The listing builds one solid part. Answer for the finished solid, in the listing's coordinates (mm). A direction names the side the tool comes from. Round coordinates to 2 decimals unless told otherwise and drop trailing zeros. Order: outer loops, then holes, each group sorted by start corner. A loop starts at its lowest first (then second) coordinate and runs counter-clockwise, first axis right, second up. Notation, with made-up numbers: (-37, -36.5) - (1, -36.5) arc R22 cw to (1, -15.5) - close; hole circle Ø8 at (15.5, 74). An arc over 180 degrees is marked (long way). Write item = value, one per line.
from build123d import *

# Parameters (mm, degrees)
F0_R     = 6.25
F1_DEPTH = 12.5
F3_DEPTH = 38
F4_R     = 18.99999
F5_R     = 2.5
F6_DEPTH = 5
F7_R     = 7.5
F8_DEPTH = 100


# Not quite as in the source:
# - a fillet or chamfer is up to 0.001 mm smaller than in the source, because OpenCascade refuses the exact size


with BuildPart() as f1:
    # F0 (on Top) → F1 (new body)
    with BuildSketch(Plane.XY):
        with BuildLine():
            Line((-13, 25.5), (-13, 0))
            ThreePointArc((-13, 0), (0, -13), (13, 0))
            Line((13, 0), (13, 13))
            Line((13, 13), (77, 13))
            Line((77, 13), (77, 0))
            ThreePointArc((77, 0), (90, -13), (103, 0))
            Line((103, 0), (103, 64))
            ThreePointArc((103, 64), (90, 77), (77, 64))
            Line((77, 64), (77, 51))
            Line((77, 51), (13, 51))
            Line((13, 51), (13, 64))
            ThreePointArc((13, 64), (0, 77), (-13, 64))
            Line((-13, 64), (-13, 38.5))
            Line((-13, 38.5), (0, 38.5))
            ThreePointArc((0, 38.5), (6.5, 32), (0, 25.5))
            Line((0, 25.5), (-13, 25.5))
        make_face()
        Circle(F0_R, mode=Mode.SUBTRACT)
        with Locations((90, 0)):
            Circle(F0_R, mode=Mode.SUBTRACT)
        with Locations((0, 64)):
            Circle(F0_R, mode=Mode.SUBTRACT)
        with Locations((90, 64)):
            Circle(F0_R, mode=Mode.SUBTRACT)
    extrude(amount=F1_DEPTH)

    # F2 (on face) → F3 (join)
    with BuildSketch(Plane.XZ.offset(-13)):
        Polygon((26.6324676319, 12.5), (77, 12.5), (103, 12.5), (64.8162338159, 50.6837661841), align=None)
    extrude(amount=-F3_DEPTH)

    # F4 (radius 19 in the source; OpenCascade refuses exactly that, so slightly less here)
    f4_edges = [f1.edges().sort_by_distance(p)[0] for p in [
        (45.724351, 13, 31.591883),
        (45.724351, 51, 31.591883),
    ]]
    fillet(f4_edges, radius=F4_R)

    # F5 (on face) → F6 (cut)
    with BuildSketch(Plane(origin=(57.75, 0, 57.75), x_dir=(0.7071067812, 0, -0.7071067812), z_dir=(0.7071067812, 0, 0.7071067812))):
        with Locations((25.1304512677, 20.1117935463)):
            Circle(F5_R)
        with Locations((39.1058761271, 24.6526843463)):
            Circle(F5_R)
        with Locations((39.1058761271, 39.3473156537)):
            Circle(F5_R)
        with Locations((25.1304512677, 43.8882064537)):
            Circle(F5_R)
        with Locations((16.4931636974, 32)):
            Circle(F5_R)
    extrude(amount=-F6_DEPTH, mode=Mode.SUBTRACT)

    # F7 (on face) → F8 (cut)
    with BuildSketch(Plane(origin=(57.75, 0, 57.75), x_dir=(0.7071067812, 0, -0.7071067812), z_dir=(0.7071067812, 0, 0.7071067812))):
        with Locations((28.9931636974, 32)):
            Circle(F7_R)
    extrude(amount=-F8_DEPTH, mode=Mode.SUBTRACT)


solid = f1.part
Q1. For faces 1 (the face through (13, 57, 6)), 2 (the face through (81.84, 39.38, 26.59)), 3 (the face through (6.5, 32.1, 6.2)), determine the directions among +Z, -Z, +X, -X, +Y, -Y from which every point of the face is accessible in a straight line to the end or side of a thin tool.
Model answer:
face_1 = +Z, -Z, +Y
face_2 = none
face_3 = +Z, -Z, -X
Q2. Section B-B on x = 90 is taken. Determine the outline of the cut face in (y, z), then the cut area to 3 significant figures.
Model answer:
outline = (-13, 0) - (-6.25, 0) - (-6.25, 12.5) - (-13, 12.5) - close; (6.25, 0) - (57.75, 0) - (57.75, 12.5) - (51, 12.5) - (51, 25.5) - (13, 25.5) - (13, 12.5) - (6.25, 12.5) - close; (70.25, 0) - (77, 0) - (77, 12.5) - (70.25, 12.5) - close
area = 1,310 mm^2
Q3. Section D-D on x = 24 is taken. Determine the outline of the cut face in (y, z).
Model answer:
outline = (13, 0) - (51, 0) - (51, 12.5) - (13, 12.5) - close
Q4. Section A-A on y = 54.5 is taken. Determine the outline of the cut face in (x, z).
Model answer:
outline = (-13, 0) - (13, 0) - (13, 12.5) - (-13, 12.5) - close; (77, 0) - (103, 0) - (103, 12.5) - (77, 12.5) - close
Q5. Find the intervals of material crossed by line 1 (Y direction, x = 90, z = 6.75); line 2 (X direction, y = 53, z = 3); line 3 (Z direction, x = 91, y = 22), in increasing order. Write a range as from..to.
Model answer:
line_1 = -13..-6.25, 6.25..57.75, 70.25..77
line_2 = -13..13, 77..103
line_3 = 0..24.5
Q6. Flat-ended cylindrical pins translate along their axes: P1, Ø11, axis at x = 90, y = 0, coming from the +Z side; P2, Ø20, axis at x = 26, y = 52.5, coming from the +Z side; P3, Ø8, axis at x = 53.5, z = 41.5, coming from the -Y side; P4, Ø18.5, axis at x = 65.5, z = 11, coming from the -Y side. Find the tip coordinate at first contact, or state that the pin passes through.
Model answer:
P1 = through
P2 = 12.5
P3 = 22.59
P4 = 13
Q7. Determine the mould class of faces 4 (the face through (-13, 51, 6)), 5 (the face through (57, 51, 15)), 6 (the face through (93, 6, 12.5)) for opening direction X: released by +X, released by -X, zero draft, split by the parting line, or undercut.
Model answer:
face_4 = released by -X
face_5 = undercut
face_6 = zero draft
Q8. Section C-C on y = 1.5 is taken. Determine the outline of the cut face in (x, z), then the cut area to 3 significant figures.
Model answer:
outline = (-13, 0) - (-6.07, 0) - (-6.07, 12.5) - (-13, 12.5) - close; (6.07, 0) - (13, 0) - (13, 12.5) - (6.07, 12.5) - close; (77, 0) - (83.93, 0) - (83.93, 12.5) - (77, 12.5) - close; (96.07, 0) - (103, 0) - (103, 12.5) - (96.07, 12.5) - close
area = 347 mm^2
